Part model, mm, in its own coordinate system. A direction names the side the tool comes from. Give positions to 0.01 mm unless a question says otherwise; leave off trailing zeros. Write each loop counter-clockwise with the first axis right and the second up, starting at its lowest first coordinate (ties: lowest second). Pieces come first, ordered by that corner, then holes. Notation, with made-up numbers: (-21, 77) - (27, 77) arc R23 ccw to (27, 92) - close; hole circle Ø1 at (31, 26). An arc over 180 degrees is marked (long way). Answer as a JSON object with one key per item and string values. Group by question number.
```python
from build123d import *
from OCP.BRepFilletAPI import BRepFilletAPI_MakeFillet

# Parameters (mm, degrees)
BOSS_EXTRUDE2_DEPTH = 127
FILLET1_R1          = 1.5875
FILLET1_R2          = 1.4732
SKETCH2_R           = 2.286
CUT_EXTRUDE1_DEPTH  = 76.2
FILLET3_R           = 1.778


with BuildPart() as part:
    # Sketch1 → Boss-Extrude2 (new body)
    with BuildSketch(Plane(origin=(0, 0, 0), x_dir=(1, 0, 0), z_dir=(0, 1, 0))):
        Polygon((-28.067579909, 0), (-28.067579909, -25.4), (-15.367579909, -25.4), (-15.367579909, -16.933333333), (-22.699928279, -21.166666582), (-22.699928279, -4.233333249), (-15.367579909, -8.466666667), (-15.367579909, 0), align=None)
    extrude(amount=BOSS_EXTRUDE2_DEPTH)

    # Fillet1: one fillet with a radius per group of edges: ONE call of the kernel's fillet builder (fillet() takes one radius for all edges)
    fillet1_edges_1 = [part.edges().sort_by_distance(p)[0] for p in [
        (-19.033754094, 127, 6.349999958),
        (-22.699928279, 127, 12.699999915),
        (-19.033754094, 127, 19.049999958),
        (-15.367579909, 127, 21.166666667),
        (-15.367579909, 127, 4.233333333),
        (-21.717579909, 127, 0),
        (-28.067579909, 63.5, 0),
        (-15.367579909, 63.5, 0),
        (-21.717579909, 0, 0),
        (-15.367579909, 0, 4.233333333),
        (-15.367579909, 63.5, 8.466666667),
        (-15.367579909, 63.5, 16.933333333),
        (-15.367579909, 0, 21.166666667),
        (-15.367579909, 63.5, 25.4),
        (-22.699928279, 0, 12.699999915),
        (-28.067579909, 127, 12.7),
        (-21.717579909, 127, 25.4),
        (-28.067579909, 63.5, 25.4),
        (-28.067579909, 0, 12.7),
        (-21.717579909, 0, 25.4),
        (-19.033754094, 0, 6.349999958),
        (-19.033754094, 0, 19.049999958),
    ]]
    fillet1_edges_2 = [part.edges().sort_by_distance(p)[0] for p in [
        (-22.699928279, 63.5, 4.233333249),
        (-22.699928279, 63.5, 21.166666582),
    ]]
    fillet1 = BRepFilletAPI_MakeFillet(part.part.solid().wrapped)
    for e in fillet1_edges_1:
        fillet1.Add(FILLET1_R1, e.wrapped)
    for e in fillet1_edges_2:
        fillet1.Add(FILLET1_R2, e.wrapped)
    add(Compound.cast(fillet1.Shape()), mode=Mode.REPLACE)

    # Sketch2 → Cut-Extrude1 (cut)
    with BuildSketch(Plane(origin=(0, 127, 0), x_dir=(1, 0, 0), z_dir=(0, 1, 0))):
        with Locations(Location((-25.235504788, -3.154170131, 0), (0, 0, 270))):
            Circle(SKETCH2_R)
        with Locations(Location((-25.235504788, -22.245829751, 0), (0, 0, 237.014036323))):
            Circle(SKETCH2_R)
    extrude(amount=-CUT_EXTRUDE1_DEPTH, mode=Mode.SUBTRACT)

    # Fillet3
    fillet3_edges = [part.edges().sort_by_distance(p)[0] for p in [
        (-23.990929667, 50.8, 20.328323879),
        (-25.235504788, 50.8, 0.868170131),
    ]]
    fillet(fillet3_edges, radius=FILLET3_R)


solid = part.part
```
1) Drop flat-ended pins along their axis: P1, Ø1.1, axis at x = -25.5, z = 3, coming from the +Y side; P2, Ø2.5, axis at x = -25.24, z = 3.15, coming from the +Y side; P3, Ø3.5, axis at y = 50, z = 12.5, coming from the +X side. Give the stop position or say it passes through.
2) Two-plate mould, pull along X, no slides. Class faces 1 (the cylindrical face through (-16.14, 64.37, 18.32)), 2 (the flat face through (-15.368, 63, 22)), 3 (the flat face through (-25, 0, 13)): +X half, -X half, draft (parallel to the pull), parting line (faces both ways), or undercut.
3) Saw through at C-C (y = 95). List the corners of the cut face in (x, z) (1 decimal), and give its area (3 significant figures).
4) Saw through at B-B (z = 13.5). List the corners of the cut face in (x, y) (1 decimal), and give its area (3 significant figures).
5) Which spindle directions (+Z, -Z, +X, -X, +Y, -Y) get a long thin tool onto all of the face, cutting with end or side? Do faces 4 (the flat face through (-22, 63, 0)), 5 (the flat face through (-19.1, 62.63, 19.09)), 6 (the cylindrical face through (-25.847, 90.31, 24.449)), 7 (the cylindrical face through (-18.874, 0.477, 5.92)). Say none if no direction does.
6) Saw through at A-A (y = 28.5). List the corners of the cut face in (x, z) (1 decimal), and give its area (3 significant figures).
7) Drill centre lines: line 1 along Z through (x, y) = (-22.25, 72.5); line 2 along Z through (x, y) = (-21, 71.5); line 3 along X through (y, z) = (98, 3). Where is each one in solid material? Low to high. Write a range as from..to.
Checks:
{
 "1": {"P1": "y = 50.83", "P2": "y = 50.97", "P3": "x = -22.7"},
 "2": {"face 1": "undercut", "face 2": "+X half", "face 3": "draft"},
 "3": {"outline": "(-28.1, 1.6) arc R1.6 ccw to (-26.5, 0) - (-17, 0) arc R1.6 ccw to (-15.4, 1.6) - (-15.4, 5.7) arc R1.6 ccw to (-17.7, 7.1) - (-20.5, 5.5) arc R1.5 cw to (-22.7, 6.8) - (-22.7, 18.6) arc R1.5 cw to (-20.5, 19.9) - (-17.7, 18.3) arc R1.6 ccw to (-15.4, 19.7) - (-15.4, 23.8) arc R1.6 ccw to (-17, 25.4) - (-26.5, 25.4) arc R1.6 ccw to (-28.1, 23.8) - close; hole circle Ø4.6 at (-25.2, 3.2); hole circle Ø4.6 at (-25.2, 22.2)", "area": "194 mm2"},
 "4": {"outline": "(-28.1, 1.6) arc R1.6 ccw to (-26.5, 0) - (-24.3, 0) arc R1.6 ccw to (-22.7, 1.6) - (-22.7, 125.4) arc R1.6 ccw to (-24.3, 127) - (-26.5, 127) arc R1.6 ccw to (-28.1, 125.4) - close", "area": "680 mm2"},
 "5": {"face 4": "-Z, +X, -X, +Y, -Y", "face 5": "+Y, -Y", "face 6": "+Y", "face 7": "-Y"},
 "6": {"outline": "(-28.1, 1.6) arc R1.6 ccw to (-26.5, 0) - (-17, 0) arc R1.6 ccw to (-15.4, 1.6) - (-15.4, 5.7) arc R1.6 ccw to (-17.7, 7.1) - (-20.5, 5.5) arc R1.5 cw to (-22.7, 6.8) - (-22.7, 18.6) arc R1.5 cw to (-20.5, 19.9) - (-17.7, 18.3) arc R1.6 ccw to (-15.4, 19.7) - (-15.4, 23.8) arc R1.6 ccw to (-17, 25.4) - (-26.5, 25.4) arc R1.6 ccw to (-28.1, 23.8) - close", "area": "227 mm2"},
 "7": {"line 1": "0..5.73, 19.67..25.4", "line 2": "0..5.33, 20.07..25.4", "line 3": "-28.07..-27.52, -22.95..-15.37"}
}
